Part model, mm, in its own coordinate system. Face numbers are marked on the shaded views. A direction names the side the tool comes from. Round coordinates to 2 decimals unless told otherwise and drop trailing zeros. Loops run counter-clockwise (first coordinate to the right, second up) from the corner with the lowest first, then second, coordinate; pieces in that order, holes last. Notation, with made-up numbers: (-29, 71.25) -> (-18, 71.25) arc R20 ccw to (-18, 98.25) -> close; hole circle Ø9 at (44, 33.25). An arc over 180 degrees is marked (long way). Answer as a JSON object with one key per item and string values. Group by question number.
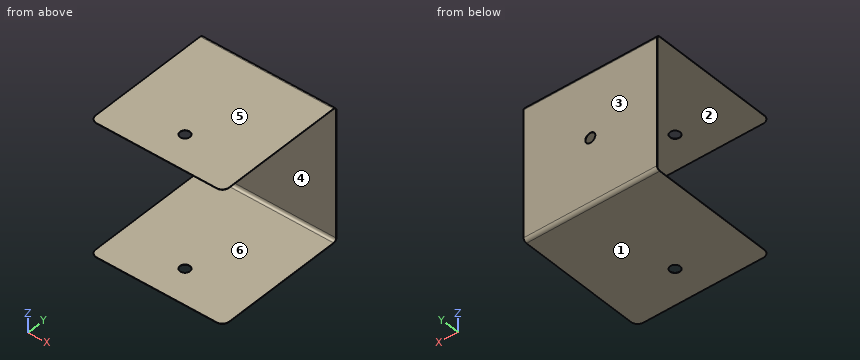
Autodesk Inventor part; units mm, degrees
ref_plane "Work Plane1" through (0, -20, 20) normal (0, 1, 0) x (-1, 0, 0)
ref_plane "YZ Plane" through (0, 0, 0) normal (1, 0, 0) x (0, 1, 0)
ref_plane "XY Plane" through (0, 0, 0) normal (0, 0, 1) x (1, 0, 0)
sketch "Sketch1" plane through (0, 0, 0) normal (1, 0, 0) x (0, 1, 0)
  line L0 (20, 20) -> (-20, 20) construction
  line L1 (-20, 20) -> (-20, -20) construction
  line L2 (-20, -20) -> (20, -20) construction
  line L3 (20, -20) -> (20, 20) construction
  line L4 (20, 20) -> (-20, -20) construction
  line L5 (-20, 20) -> (20, -20) construction
  line L6 (-20, 20) -> (19, 20)
  arc A0 (20, 19) -> (19, 20) centre (19, 19) ccw
  line L7 (-20, -20) -> (19, -20)
  arc A1 (19, -20) -> (20, -19) centre (19, -19) ccw
  line L8 (20, -19) -> (20, 19)
  point P0 (0, 0)
  dimension "d0" = 40
  dimension "d1" = 40
  dimension "d2" = 39
  dimension "d3" = 39
ref_plane "Work Plane1" through (0, -20, 20) normal (0, 1, 0) x (-1, 0, 0)
sketch "Sketch2" plane through (0, -20, 20) normal (0, 1, 0) x (-1, 0, 0)
  line L0 (0, 0) -> (40, 0)
  line L1 (40, 0) -> (40, -0.1)
  line L2 (40, -0.1) -> (0, -0.1)
  line L3 (0, -0.1) -> (0, 0)
  point P0 (0, -20)
  dimension "d4" = 40
  dimension "d5" = 0.1
sweep "Sweep1" add profiles "Sketch2" path "Sketch1"
fillet "Fillet1" radius 2 4 edges at (0, -20, 19.95) (0, -20, -19.95) (-40, -20, 19.95) (-40, -20, -19.95)
sketch "Sketch3" plane through (-40, 19, 20) normal (0, 0, 1) x (1, 0, 0)
  circle A0 centre (20, -29) radius 1.5
  line L0 (0, 0) -> (0, -37) construction
  line L1 (0, -29) -> (40, -29) construction
  line L2 (40, 0) -> (40, -37) construction
  line L3 (38, -39) -> (2, -39) construction
  point P0 (40, -19)
  dimension "d9" = 3
  dimension "d10" = 10
  dimension "d11" = 20
extrude "Extrusion1" cut sketch "Sketch3" against normal through all
surface extrude "ExtrusionSrf1" sketch "Sketch3" against normal through all shown yes curves A0
sketch "Sketch4" plane through (-40, 20, 19) normal (0, 1, 0) x (1, 0, 0)
  line L0 (0, 0) -> (40, 0) construction
  line L1 (0, 38) -> (40, 38) construction
  line L2 (0, 0) -> (40, 38) construction
  line L3 (40, 0) -> (40, 38) construction
  line L4 (40, 0) -> (0, 38) construction
  point P0 (40, 19)
  point P1 (20, 19)
hole "Hole1" at (-20, 20, 0) direction (0, -1, 0) diameter 3 end through all
equation "\"d3\" = d2"
properties material "Iron, Malleable"
Item 1: Drop a flat-ended pin along its axis: pin 1 Ø5 at (x, z) = (-20, 0) entering from +Y. Give the stop position or say it passes through.
Item 2: Band-saw the part on A-A, the plane z = 0. List the corners of the cut face in (x, y), plus the area to 3 significant figures.
Item 3: Two-plate mould, pull along Z, no slides. Class the marked faces 1, 2, 3 and 4: pulls with the +Z half, pulls with the -Z half, needs draft (parallel to the pull), parting line crosses it, or undercut.
Item 4: Band-saw the part on D-D, the plane x = -11.5. List the corners of the cut face in (y, z), plus the area to 3 significant figures.
Item 5: Band-saw the part on B-B, the plane x = -20. List the corners of the cut face in (y, z), plus the area to 3 significant figures.
Item 6: Band-saw the part on C-C, the plane y = -10. List the corners of the cut face in (x, z).
Item 7: Which spindle directions (+Z, -Z, +X, -X, +Y, -Y) get a long thin tool onto all of the face, cutting with end or side? Do the marked faces 5 and 6. Say none if no direction does.
Entries:
{
 "1": {"pin 1": "y = 20"},
 "2": {"outline": "(-40, 19.9) -> (-21.5, 19.9) -> (-21.5, 20) -> (-40, 20) -> close; (-18.5, 19.9) -> (0, 19.9) -> (0, 20) -> (-18.5, 20) -> close", "area": "3.70 mm²"},
 "3": {"face 1": "pulls with the -Z half", "face 2": "undercut", "face 3": "needs draft", "face 4": "undercut"},
 "4": {"outline": "(-20, -20) -> (19, -20) arc R1 ccw to (20, -19) -> (20, 19) arc R1 ccw to (19, 20) -> (-20, 20) -> (-20, 19.9) -> (19, 19.9) arc R0.9 cw to (19.9, 19) -> (19.9, -19) arc R0.9 cw to (19, -19.9) -> (-20, -19.9) -> close", "area": "11.9 mm²"},
 "5": {"outline": "(-20, -20) -> (-11.5, -20) -> (-11.5, -19.9) -> (-20, -19.9) -> close; (-20, 19.9) -> (-11.5, 19.9) -> (-11.5, 20) -> (-20, 20) -> close; (-8.5, -20) -> (19, -20) arc R1 ccw to (20, -19) -> (20, -1.5) -> (19.9, -1.5) -> (19.9, -19) arc R0.9 cw to (19, -19.9) -> (-8.5, -19.9) -> close; (-8.5, 19.9) -> (19, 19.9) arc R0.9 cw to (19.9, 19) -> (19.9, 1.5) -> (20, 1.5) -> (20, 19) arc R1 ccw to (19, 20) -> (-8.5, 20) -> close", "area": "11.0 mm²"},
 "6": {"outline": "(-40, -20) -> (-21.5, -20) -> (-21.5, -19.9) -> (-40, -19.9) -> close; (-40, 19.9) -> (-21.5, 19.9) -> (-21.5, 20) -> (-40, 20) -> close; (-18.5, -20) -> (0, -20) -> (0, -19.9) -> (-18.5, -19.9) -> close; (-18.5, 19.9) -> (0, 19.9) -> (0, 20) -> (-18.5, 20) -> close"},
 "7": {"face 5": "+Z, +X, -X, +Y, -Y", "face 6": "+X, -X, -Y"}
}
